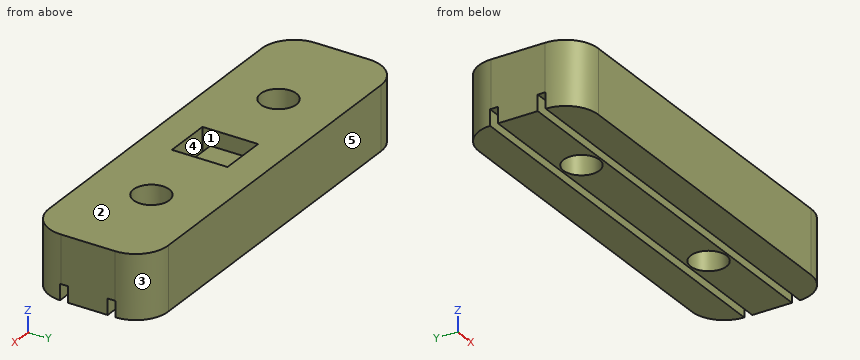
```python
from build123d import *

# Parameters (mm, degrees)
F0_W     = 22
F0_H     = 1
F0_H_2   = 5
F1_DEPTH = 8
F0_W_2   = 6
F2_DEPTH = 17.526
F3_D     = 4.5
F3_DEPTH = 10
F4_DEPTH = 6
F5_DEPTH = 2
F6_R     = 4.0894


with BuildPart() as f1:
    # F0 (on Top) → F1 (new body)
    with BuildSketch(Plane.XY):
        Polygon((25, 3.5), (25, 7.5), (-25, 7.5), (-25, 3.5), (-3, 3.5), (3, 3.5), align=None)
        with Locations((14, -3)):
            Rectangle(F0_W, F0_H)
        with Locations((-14, -3)):
            Rectangle(F0_W, F0_H)
        Polygon((25, -7.5), (25, -3.5), (3, -3.5), (-3, -3.5), (-25, -3.5), (-25, -7.5), align=None)
        with Locations((-14, 0)):
            Rectangle(F0_W, F0_H_2)
        with Locations((14, 0)):
            Rectangle(F0_W, F0_H_2)
        with Locations((14, 3)):
            Rectangle(F0_W, F0_H)
        with Locations((-14, 3)):
            Rectangle(F0_W, F0_H)
    extrude(amount=F1_DEPTH)

    # F0 (on Top) → F2 (cut)
    with BuildSketch(Plane.XY):
        with Locations((0, 3)):
            Rectangle(F0_W_2, F0_H)
    extrude(amount=F2_DEPTH, mode=Mode.SUBTRACT)

    # F3
    with Locations(Plane(origin=(0, 0, 0), x_dir=(1, 0, 0), z_dir=(0, 0, -1))):
        with Locations((-12.5, 0), (12.5, 0)):
            Hole(F3_D / 2, depth=F3_DEPTH)

    # F0 (on Top) → F4 (join)
    with BuildSketch(Plane.XY):
        Rectangle(F0_W_2, F0_H_2)
    extrude(amount=F4_DEPTH)

    # F0 (on Top) → F5 (cut)
    with BuildSketch(Plane.XY):
        with Locations((-14, -3)):
            Rectangle(F0_W, F0_H)
        with Locations((14, -3)):
            Rectangle(F0_W, F0_H)
        with Locations((14, 3)):
            Rectangle(F0_W, F0_H)
        with Locations((-14, 3)):
            Rectangle(F0_W, F0_H)
    extrude(amount=F5_DEPTH, mode=Mode.SUBTRACT)

    # F6
    f6_edges = [f1.edges().sort_by_distance(p)[0] for p in [
        (25, -7.5, 4),
        (25, 7.5, 4),
        (-25, 7.5, 4),
        (-25, -7.5, 4),
    ]]
    fillet(f6_edges, radius=F6_R)


solid = f1.part
```
CAD build for the part. Positions are in the model's coordinates, mm. Face numbers are marked on the shaded views. A direction names the side the tool comes from. Give positions to 0.01 mm unless a question says otherwise; leave off trailing zeros. Write each loop counter-clockwise with the first axis right and the second up, starting at its lowest first coordinate (ties: lowest second). Pieces come first, ordered by that corner, then holes. Notation, with made-up numbers: (32.25, 11) -> (53.25, 11) arc R22 ccw to (53.25, 41) -> close; hole circle Ø7 at (49.5, 41). An arc over 180 degrees is marked (long way). Write each question's results on one line, items separated by ' | '.
1. Cut at B-B, the plane x = -12.5. Write the cut outline in (y, z), then the cut area to 3 significant figures.
Geometry check:
outline: (-7.5, 0) -> (-3.5, 0) -> (-3.5, 2) -> (-2.5, 2) -> (-2.5, 0) -> (-2.25, 0) -> (-2.25, 8) -> (-7.5, 8) -> close; (2.25, 0) -> (2.5, 0) -> (2.5, 2) -> (3.5, 2) -> (3.5, 0) -> (7.5, 0) -> (7.5, 8) -> (2.25, 8) -> close | area: 80.0 mm²
2. Wall check: probe 1 along Y at (x, z) = (1, 2.25); probe 2 along Y at (x, z) = (-12.5, 3.5); probe 3 along X at (y, z) = (-0.75, 0.5). Give the ranges that are in metal, low to high. Write a range as [from, to].
Geometry check:
probe 1: [-7.5, -3.5], [-2.5, 2.5], [3.5, 7.5] | probe 2: [-7.5, -2.25], [2.25, 7.5] | probe 3: [-25, -14.62], [-10.38, 10.38], [14.62, 25]
3. Cut at A-A, the plane z = 4.25. Write the cut outline in (x, y).
Geometry check:
outline: (-25, -3.41) arc R4.09 ccw to (-20.91, -7.5) -> (20.91, -7.5) arc R4.09 ccw to (25, -3.41) -> (25, 3.41) arc R4.09 ccw to (20.91, 7.5) -> (-20.91, 7.5) arc R4.09 ccw to (-25, 3.41) -> close; hole circle Ø4.5 at (-12.5, 0); hole (-3, -3.5) -> (3, -3.5) -> (3, -2.5) -> (-3, -2.5) -> close; hole (-3, 2.5) -> (3, 2.5) -> (3, 3.5) -> (-3, 3.5) -> close; hole circle Ø4.5 at (12.5, 0)
4. Which spindle directions (+Z, -Z, +X, -X, +Y, -Y) get a long thin tool onto all of the face, cutting with end or side? Do the marked faces 4 and 5. Say none if no direction does.
Geometry check:
face 4: -Z | face 5: +Z, -Z, +X, -X, +Y
5. Cut at C-C, the plane z = 0.5. Write the cut outline in (x, y), then the cut area to 3 significant figures.
Geometry check:
outline: (-25, -3.5) arc R4.09 ccw to (-20.91, -7.5) -> (20.91, -7.5) arc R4.09 ccw to (25, -3.5) -> close; (-25, -2.5) -> (25, -2.5) -> (25, 2.5) -> (-25, 2.5) -> close; (-25, 3.5) -> (25, 3.5) arc R4.09 ccw to (20.91, 7.5) -> (-20.91, 7.5) arc R4.09 ccw to start; hole circle Ø4.5 at (-12.5, 0); hole circle Ø4.5 at (12.5, 0) | area: 604 mm²
6. Cut at D-D, the plane y = 0. Write the cut outline in (x, z).
Geometry check:
outline: (-25, 0) -> (-14.75, 0) -> (-14.75, 8) -> (-25, 8) -> close; (-10.25, 0) -> (10.25, 0) -> (10.25, 8) -> (3, 8) -> (3, 6) -> (-3, 6) -> (-3, 8) -> (-10.25, 8) -> close; (14.75, 0) -> (25, 0) -> (25, 8) -> (14.75, 8) -> close
7. Two-plate mould, pull along Y, no slides. Class the marked faces 1, 2 and 3: pulls with the +Y half, pulls with the -Y half, needs draft (parallel to the pull), parting line crosses it, or undercut.
Geometry check:
face 1: undercut | face 2: needs draft | face 3: pulls with the +Y half
8. Drop flat-ended pins along their axis: P1, Ø0.5, axis at x = -15, y = -3, coming from the -Z side; P2, Ø4, axis at x = -12.5, y = 0, coming from the -Z side. Give the stop position or say it passes through.
Geometry check:
P1: z = 2 | P2: through
